from build123d import *

# Parameters (mm, degrees)
SCHIZZO2_R    = 37.5
SCHIZZO2_R_2  = 13
SCHIZZO2_R_3  = 25
SCHIZZO2_R_4  = 5
PIASTRA_DEPTH = 30


with BuildPart() as part:
    # Schizzo2 → Piastra (new body)
    with BuildSketch(Plane.XY):
        with BuildLine():
            Line((20, 215), (-20, 215))
            ThreePointArc((-20, 215), (-76.568542495, 191.568542495), (-100, 135))
            Line((-100, 135), (-100, -135))
            ThreePointArc((-100, -135), (-76.568542495, -191.568542495), (-20, -215))
            Line((-20, -215), (20, -215))
            ThreePointArc((20, -215), (76.568542495, -191.568542495), (100, -135))
            Line((100, -135), (100, 135))
            ThreePointArc((100, 135), (76.568542495, 191.568542495), (20, 215))
        make_face()
        Circle(SCHIZZO2_R, mode=Mode.SUBTRACT)
        with Locations((0, -160)):
            Circle(SCHIZZO2_R_2, mode=Mode.SUBTRACT)
        with Locations((0, 160)):
            Circle(SCHIZZO2_R_3, mode=Mode.SUBTRACT)
        with Locations((0, 55)):
            Circle(SCHIZZO2_R_4, mode=Mode.SUBTRACT)
        with Locations((0, -55)):
            Circle(SCHIZZO2_R_4, mode=Mode.SUBTRACT)
    extrude(amount=PIASTRA_DEPTH)


solid = part.part
Geometry: final body of the model. Coordinates: model frame, mm. Give positions to 0.01 mm unless a question says otherwise; leave off trailing zeros. Order: outer loops, then holes, each group sorted by start corner. A loop starts at its lowest first (then second) coordinate and runs counter-clockwise, first axis right, second up. Notation, with made-up numbers: (56.25, -23) -> (74.25, -23) arc R24 ccw to (74.25, 15) -> close; hole circle Ø1 at (-34.5, -30). An arc over 180 degrees is marked (long way). Answer as a JSON object with one key per item and string values.
Q1. Draft query along Y for faces 1 (the flat face through (0, 215, 15)), 2 (the cylindrical face through (75.94, -192.19, 14.79)), 3 (the cylindrical face through (-0.651, -50.043, 14.79)). Return one class per face: released by +Y, released by -Y, zero draft, split by the parting line, or undercut.
Entries:
{"face 1": "released by +Y", "face 2": "released by -Y", "face 3": "undercut"}
Q2. Section D-D (y = 0). Output: boundary loops of the cut face in (x, z), plus the area to 3 significant figures.
Entries:
{"outline": "(-100, 0) -> (-37.5, 0) -> (-37.5, 30) -> (-100, 30) -> close; (37.5, 0) -> (100, 0) -> (100, 30) -> (37.5, 30) -> close", "area": "3,750 mm^2"}
Q3. First-contact query: pin 1 (1.5 mm diameter, centred on y = 166, z = 17, fed in from +X); pin 2 (8 mm diameter, centred on x = -46.5, z = 11, fed in from +Y); pin 3 (6 mm diameter, centred on x = -69.5, z = 14, fed in from +Y). Flat tips, straight axial feed; report the tip coordinate or a pass-through.
Entries:
{"pin 1": "stops at x = 94.06", "pin 2": "stops at y = 211.77", "pin 3": "stops at y = 200.1"}
Q4. Section A-A (y = -55). Output: boundary loops of the cut face in (x, z).
Entries:
{"outline": "(-100, 0) -> (-5, 0) -> (-5, 30) -> (-100, 30) -> close; (5, 0) -> (100, 0) -> (100, 30) -> (5, 30) -> close"}
Q5. Section B-B (z = 24.5). Output: boundary loops of the cut face in (x, y).
Entries:
{"outline": "(-100, -135) arc R80 ccw to (-20, -215) -> (20, -215) arc R80 ccw to (100, -135) -> (100, 135) arc R80 ccw to (20, 215) -> (-20, 215) arc R80 ccw to (-100, 135) -> close; hole circle Ø75 at (0, 0); hole circle Ø50 at (0, 160); hole circle Ø26 at (0, -160); hole circle Ø10 at (0, -55); hole circle Ø10 at (0, 55)"}
Q6. Section C-C (x = 0). Output: boundary loops of the cut face in (y, z), plus the area to 3 significant figures.
Entries:
{"outline": "(-215, 0) -> (-173, 0) -> (-173, 30) -> (-215, 30) -> close; (-147, 0) -> (-60, 0) -> (-60, 30) -> (-147, 30) -> close; (-50, 0) -> (-37.5, 0) -> (-37.5, 30) -> (-50, 30) -> close; (37.5, 0) -> (50, 0) -> (50, 30) -> (37.5, 30) -> close; (60, 0) -> (135, 0) -> (135, 30) -> (60, 30) -> close; (185, 0) -> (215, 0) -> (215, 30) -> (185, 30) -> close", "area": "7,770 mm^2"}
Q7. Material intervals for probe 1 along Y at (x, z) = (0, 19); probe 2 along Y at (x, z) = (11.5, 10.5); probe 3 along Y at (x, z) = (14.5, 13.5), sorted ascending.
Entries:
{"probe 1": "y = -215 to -173, -147 to -60, -50 to -37.5, 37.5 to 50, 60 to 135, 185 to 215", "probe 2": "y = -215 to -166.06, -153.94 to -35.69, 35.69 to 137.8, 182.2 to 215", "probe 3": "y = -215 to -34.58, 34.58 to 139.63, 180.37 to 215"}
